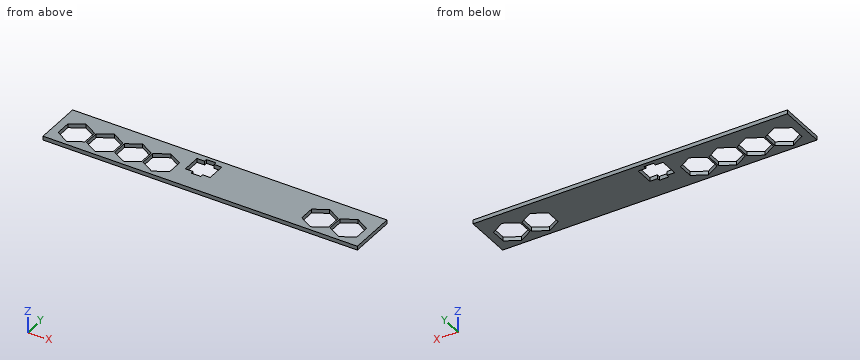
from build123d import *

# Parameters (mm, degrees)
SKETCH1_W           = 254
SKETCH1_H           = 38.1
BOSS_EXTRUDE1_DEPTH = 3.175
CUT_EXTRUDE1_DEPTH  = 10.414
CUT_EXTRUDE2_DEPTH  = 3.175


with BuildPart() as part:
    # Sketch1 → Boss-Extrude1 (new body)
    with BuildSketch(Plane.XY):
        Rectangle(SKETCH1_W, SKETCH1_H)
    extrude(amount=BOSS_EXTRUDE1_DEPTH)

    # Sketch4 → Cut-Extrude1 (cut)
    with BuildSketch(Plane.XY.offset(3.175)):
        Polygon((-99.060120052, -9.6425385), (-99.060120052, 2.8223845), (-109.855060026, 9.054846), (-120.65, 2.8223845), (-120.65, -9.6425385), (-109.855060026, -15.875), align=None)
        Polygon((-76.200120052, -9.6425385), (-76.200120052, 2.8223845), (-86.995060026, 9.054846), (-97.79, 2.8223845), (-97.79, -9.6425385), (-86.995060026, -15.875), align=None)
        Polygon((-53.340120052, -9.6425385), (-53.340120052, 2.8223845), (-64.135060026, 9.054846), (-74.93, 2.8223845), (-74.93, -9.6425385), (-64.135060026, -15.875), align=None)
        Polygon((-30.480120052, -9.6425385), (-30.480120052, 2.8223845), (-41.275060026, 9.054846), (-52.07, 2.8223845), (-52.07, -9.6425385), (-41.275060026, -15.875), align=None)
        Polygon((120.65, -9.6425385), (120.65, 2.8223845), (109.855060026, 9.054846), (99.060120052, 2.8223845), (99.060120052, -9.6425385), (109.855060026, -15.875), align=None)
        Polygon((97.79, -9.6425385), (97.79, 2.8223845), (86.995060026, 9.054846), (76.200120052, 2.8223845), (76.200120052, -9.6425385), (86.995060026, -15.875), align=None)
    extrude(amount=-CUT_EXTRUDE1_DEPTH, mode=Mode.SUBTRACT)

    # Sketch2 → Cut-Extrude2 (cut)
    with BuildSketch(Plane.XY.offset(3.175)):
        Polygon((-3.20675, -1.11125), (-3.20675, 13.81125), (-9.398, 13.81125), (-9.398, 16.1925), (-17.018, 16.1925), (-17.018, 13.81125), (-23.20925, 13.81125), (-23.20925, -1.11125), (-17.018, -1.11125), (-17.018, -3.4925), (-9.398, -3.4925), (-9.398, -1.11125), align=None)
    extrude(amount=-CUT_EXTRUDE2_DEPTH, mode=Mode.SUBTRACT)


solid = part.part
Read the model definition and answer for the solid it produces. Units are mm, in the model's axes. Coordinates: 2 decimals unless noted, no trailing zeros. Write each loop counter-clockwise with the first axis right and the second up, starting at its lowest first coordinate (ties: lowest second). Pieces come first, ordered by that corner, then holes. Notation, with made-up numbers: (12, -14.75) - (42, -14.75) arc R26 cw to (42, 12.25) - close; hole circle Ø5 at (-35, 57). An arc over 180 degrees is marked (long way). One line per question, with ' | ' between items.
Q1. Find section C-C, the plane y = 6. State how many separate pieces and enclosed holes the cut face has, plus the area to 3 significant figures.
Result set:
separate pieces: 8 | enclosed holes: 0 | area: 541 mm^2
Q2. This flat-tipped pin is pushed along its axis until it touches: P1, Ø3, axis at x = -42, y = -12.5, coming from the -Z side. Where does it stop, or does it pass through?
Result set:
P1: through
Q3. Consider L1, parallel to Y at x = -11, z = 0.6; L2, parallel to X at y = 10.5, z = 1.65; L3, parallel to Y at x = -22, z = 1.05. Determine where each line is inside the solid, lowest interval first. Write a range as [from, to].
Result set:
L1: [-19.05, -3.49], [16.19, 19.05] | L2: [-127, -23.21], [-3.21, 127] | L3: [-19.05, -1.11], [13.81, 19.05]
Q4. Find section B-B, the plane x = -6. Write down the section's boundary in (y, z) (3 decimals).
Result set:
outline: (-19.05, 0) - (-1.111, 0) - (-1.111, 3.175) - (-19.05, 3.175) - close; (13.811, 0) - (19.05, 0) - (19.05, 3.175) - (13.811, 3.175) - close
Q5. Find section A-A, the plane y = -7.5. Write down the section's boundary in (x, z) (3 decimals).
Result set:
outline: (-127, 0) - (-120.65, 0) - (-120.65, 3.175) - (-127, 3.175) - close; (-99.06, 0) - (-97.79, 0) - (-97.79, 3.175) - (-99.06, 3.175) - close; (-76.2, 0) - (-74.93, 0) - (-74.93, 3.175) - (-76.2, 3.175) - close; (-53.34, 0) - (-52.07, 0) - (-52.07, 3.175) - (-53.34, 3.175) - close; (-30.48, 0) - (76.2, 0) - (76.2, 3.175) - (-30.48, 3.175) - close; (97.79, 0) - (99.06, 0) - (99.06, 3.175) - (97.79, 3.175) - close; (120.65, 0) - (127, 0) - (127, 3.175) - (120.65, 3.175) - close
